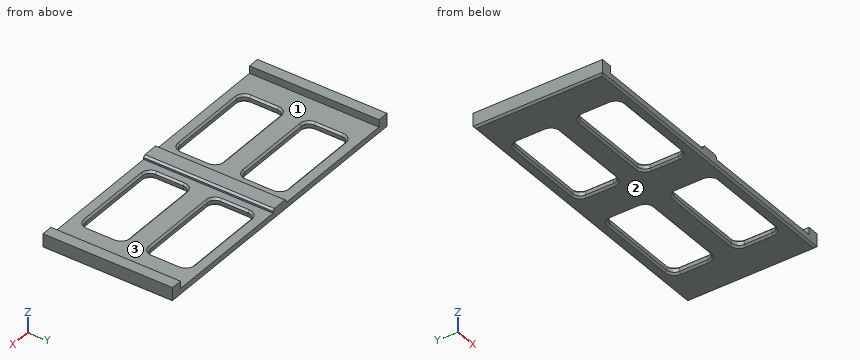
from build123d import *

# Parameters (mm, degrees)
F0_W     = 81
F0_H     = 35
F1_DEPTH = 2
F2_W     = 5
F2_H     = 35
F3_DEPTH = 1
F4_W     = 3
F4_H     = 35
F5_DEPTH = 2
F7_DEPTH = 2.001
F8_SIZE  = 0.5
F9_SIZE  = 0.5


with BuildPart() as f1:
    # F0 (on Top) → F1 (new body)
    with BuildSketch(Plane.XY):
        Rectangle(F0_W, F0_H)
    extrude(amount=F1_DEPTH)

    # F2 (on face) → F3 (join)
    with BuildSketch(Plane.XY.offset(2)):
        Rectangle(F2_W, F2_H)
    extrude(amount=F3_DEPTH)

    # F4 (on face) → F5 (join)
    with BuildSketch(Plane.XY.offset(2)):
        with Locations((-39, 0)):
            Rectangle(F4_W, F4_H)
        with Locations((39, 0)):
            Rectangle(F4_W, F4_H)
    extrude(amount=F5_DEPTH)

    # F6 (on face) → F7 (cut, through all)
    with BuildSketch(Plane.XY.offset(2)):
        with BuildLine():
            Line((-7, 14.5), (-28.5, 14.5))
            ThreePointArc((-28.5, 14.5), (-29.914214, 13.914214), (-30.5, 12.5))
            Line((-30.5, 12.5), (-30.5, 5))
            ThreePointArc((-30.5, 5), (-29.914214, 3.585786), (-28.5, 3))
            Line((-28.5, 3), (-7, 3))
            ThreePointArc((-7, 3), (-5.585786, 3.585786), (-5, 5))
            Line((-5, 5), (-5, 12.5))
            ThreePointArc((-5, 12.5), (-5.585786, 13.914214), (-7, 14.5))
        make_face()
        with BuildLine():
            Line((-30.5, -5), (-30.5, -12.5))
            ThreePointArc((-30.5, -12.5), (-29.914214, -13.914214), (-28.5, -14.5))
            Line((-28.5, -14.5), (-7, -14.5))
            ThreePointArc((-7, -14.5), (-5.585786, -13.914214), (-5, -12.5))
            Line((-5, -12.5), (-5, -5))
            ThreePointArc((-5, -5), (-5.585786, -3.585786), (-7, -3))
            Line((-7, -3), (-28.5, -3))
            ThreePointArc((-28.5, -3), (-29.914214, -3.585786), (-30.5, -5))
        make_face()
        with BuildLine():
            ThreePointArc((7, 14.5), (5.585786, 13.914214), (5, 12.5))
            Line((5, 12.5), (5, 5))
            ThreePointArc((5, 5), (5.585786, 3.585786), (7, 3))
            Line((7, 3), (28.5, 3))
            ThreePointArc((28.5, 3), (29.914214, 3.585786), (30.5, 5))
            Line((30.5, 5), (30.5, 12.5))
            ThreePointArc((30.5, 12.5), (29.914214, 13.914214), (28.5, 14.5))
            Line((28.5, 14.5), (7, 14.5))
        make_face()
        with BuildLine():
            Line((28.5, -3), (7, -3))
            ThreePointArc((7, -3), (5.585786, -3.585786), (5, -5))
            Line((5, -5), (5, -12.5))
            ThreePointArc((5, -12.5), (5.585786, -13.914214), (7, -14.5))
            Line((7, -14.5), (28.5, -14.5))
            ThreePointArc((28.5, -14.5), (29.914214, -13.914214), (30.5, -12.5))
            Line((30.5, -12.5), (30.5, -5))
            ThreePointArc((30.5, -5), (29.914214, -3.585786), (28.5, -3))
        make_face()
    extrude(amount=-F7_DEPTH, mode=Mode.SUBTRACT)

    # F8
    f8_edges = [f1.edges().sort_by_distance(p)[0] for p in [
        (0, -17.5, 0),
        (40.5, 0, 0),
        (0, 17.5, 0),
        (-40.5, 0, 0),
    ]]
    chamfer(f8_edges, length=F8_SIZE)

    # F9
    f9_edges = [f1.edges().sort_by_distance(p)[0] for p in [
        (2.5, 0, 3),
        (-2.5, 0, 3),
        (17.75, -14.5, 2),
        (17.75, 3, 2),
        (-17.75, -3, 2),
        (-17.75, 3, 2),
        (-17.75, -3, 0),
        (-17.75, 14.5, 0),
        (17.75, 14.5, 0),
        (17.75, -3, 0),
    ]]
    chamfer(f9_edges, length=F9_SIZE)


solid = f1.part
Input: part model. Units: mm. Frame: model coordinates. Face numbers are marked on the shaded views. Round coordinates to 2 decimals unless told otherwise and drop trailing zeros. Write each loop counter-clockwise with the first axis right and the second up, starting at its lowest first coordinate (ties: lowest second). Pieces come first, ordered by that corner, then holes.
1) Cut plane A-A (x = 10). Return the cut outline in (y, z).
2) Ray query, L1, parallel to X at y = 10.5, z = 2.45; L2, parallel to X at y = 11, z = 1.05; L3, parallel to X at y = -3, z = 3.15. Return the intervals inside material, ascending.
3) Draft query along X for the marked faces 1, 2 and 3. Return one class per face: pulls with the +X half, pulls with the -X half, needs draft (parallel to the pull), parting line crosses it, or undercut.
4) Cut plane C-C (y = 1). Return the cut outline in (x, z).
5) Cut plane D-D (x = -3.5). Return the cut outline in (y, z), then the cut area to 4 significant figures.
6) Contact query for flat-ended pins moving along their axis: P1, Ø17.5, axis at x = 12, y = 4.5, coming from the +Z side; P2, Ø1, axis at x = -5.5, y = -4, coming from the -Z side; P3, Ø2, axis at x = -0.5, y = -3.5, coming from the +Z side. Output: stop coordinate, or through.
7) Cut plane B-B (y = 10). Count the separate pieces of the cut face and the enclosed holes in it, then the cut area to 3 significant figures.
Geometry says:
1. outline: (-17.5, 0.5) - (-17, 0) - (-15, 0) - (-14.5, 0.5) - (-14.5, 1.5) - (-15, 2) - (-17.5, 2) - close; (-3, 0.5) - (-2.5, 0) - (2.5, 0) - (3, 0.5) - (3, 1.5) - (2.5, 2) - (-2.5, 2) - (-3, 1.5) - close; (14.5, 0.5) - (15, 0) - (17, 0) - (17.5, 0.5) - (17.5, 2) - (15, 2) - (14.5, 1.5) - close
2. L1: x = -40.5 to -37.5, -2.5 to 2.5, 37.5 to 40.5
2. L2: x = -40.5 to -30.5, -5 to 5, 30.5 to 40.5
2. L3: x = -40.5 to -37.5, 37.5 to 40.5
3. face 1: undercut
3. face 2: needs draft
3. face 3: undercut
4. outline: (-40.5, 0.5) - (-40, 0) - (40, 0) - (40.5, 0.5) - (40.5, 4) - (37.5, 4) - (37.5, 2) - (2.5, 2) - (2.5, 2.5) - (2, 3) - (-2, 3) - (-2.5, 2.5) - (-2.5, 2) - (-37.5, 2) - (-37.5, 4) - (-40.5, 4) - close
5. outline: (-17.5, 0.5) - (-17, 0) - (17, 0) - (17.5, 0.5) - (17.5, 2) - (-17.5, 2) - close
5. area: 69.75 mm2
6. P1: stops at z = 2
6. P2: stops at z = 0.2
6. P3: stops at z = 3
7. separate pieces: 3
7. enclosed holes: 0
7. area: 75.5 mm2
